Autodesk Inventor part; units mm, degrees
ref_plane "YZ Plane" through (0, 0, 0) normal (1, 0, 0) x (0, 1, 0)
ref_plane "XZ Plane" through (0, 0, 0) normal (0, 1, 0) x (-1, 0, 0)
ref_plane "XY Plane" through (0, 0, 0) normal (0, 0, 1) x (1, 0, 0)
sketch "Эскиз1" plane through (0, 0, 0) normal (0, 0, 1) x (1, 0, 0)
  line L0 (-5, -1.0438) -> (49.0851, -1.0438)
  circle A0 centre (141.53, 31.3) radius 1.6
  circle A1 centre (141.53, 31.3) radius 12.8551
  line L1 (141.53, 31.3) -> (144.3584, 34.1284)
  line L2 (144.3584, 34.1284) -> (153.4483, 25.0385)
  line L3 (144.3584, 34.1284) -> (135.2685, 43.2183)
  line L4 (135.2685, 43.2183) -> (132.4401, 40.3899)
  line L5 (133.8543, 41.8041) -> (152.0341, 23.6243)
  line L6 (152.0341, 23.6243) -> (153.4483, 25.0385)
  circle A2 centre (141.53, 31.3) radius 3.5
  line L7 (133.8543, 41.8041) -> (138.2527, 30.0714)
  line L8 (141.53, 31.3) -> (150.6199, 22.2101)
  line L9 (150.6199, 22.2101) -> (153.4483, 19.3817)
  circle A3 centre (153.4483, 19.3817) radius 1.6
  circle A4 centre (153.4483, 19.3817) radius 3.5
  line L10 (139.0551, 28.8251) -> (150.9734, 16.9068)
  line L11 (153.4483, 25.0385) -> (156.198, 21.5472)
  ellipse E0 centre (50.75, 20.1064) end of major axis (50.75, -5.3184) minor radius 3 (49.0851, -1.0438) -> (50.4608, -5.2) ccw
  line L12 (-5, -9.3562) -> (-5, -1.0438)
  line L13 (49.0851, -9.3562) -> (-5, -9.3562)
  ellipse E1 centre (50.75, -30.5064) end of major axis (50.75, -5.0816) minor radius 3 (50.4608, -5.2) -> (49.0851, -9.3562) ccw
  line L14 (135.2688, -53.6185) -> (153.4482, -35.4383)
  line L15 (153.4482, -35.4383) -> (156.1979, -31.9467)
  arc A5 (156.1979, -31.9467) -> (150.9733, -27.3065) centre (153.4482, -29.7813) ccw
  line L16 (150.9733, -27.3065) -> (139.0551, -39.2252)
  arc A6 (139.0551, -39.2252) -> (138.2526, -40.4715) centre (141.5299, -41.7001) ccw
  line L17 (138.2526, -40.4715) -> (133.8546, -52.2043)
  line L18 (133.8546, -52.2043) -> (135.2688, -53.6185)
  circle A7 centre (153.4482, -29.7813) radius 1.6
  circle A8 centre (141.5299, -41.7001) radius 1.6
  arc A9 (133.5218, -22.9864) -> (138.03, -21.6481) centre (141.53, -41.7) ccw
  arc A10 (138.03, -25.2121) -> (137.4201, -25.3535) centre (141.5299, -41.7001) ccw
  line L19 (137.4201, -25.3535) -> (133.5218, -22.9864)
  line L20 (138.03, -21.6481) -> (138.03, -25.2121)
  point P0 (0, 0)
  point P1 (139.0604, -39.2199)
  point P2 (144.9752, 30.6832)
  point P3 (140.9132, 34.7452)
  point P4 (133.9107, 41.6537)
  point P5 (135.7198, 42.7671)
  dimension "d0" = 3.2
  dimension "d1" = 4
  dimension "d2" = 7
  dimension "d3" = 4
  dimension "d4" = 3.2
  dimension "d5" = 7
extrude "Выдавливание1" add sketch "Эскиз1" against normal blind 12 contours A0 L1 L5 A2 L8 | A0 L8 A2 L5 L1 | L5 A2 L1 | L1 A2 L5 | L8 A1 L10 A2 | A2 L5 A1 L8 | A2 L5 A1 L3 L1 | L1 L2 A1 L5 A2 | A2 L7 A1 L5 | L9 A4 L10 A1 | A1 L5 L6 L11 A4 L9 | L5 L4 L3 A1 | A1 L7 L5 | A1 L2 L6 L5 | A4
chamfer "Фаска1" distance 1 angle 45 2 edges at (151.8483, 19.3817, -12) (139.93, 31.3, -12)
sketch "Эскиз2" plane through (153.4483, 25.0385, 0) normal (0.7071068, 0.7071068, 0) x (0, 0, -1)
  line L0 (0, 25.7101) -> (12, 25.7101)
  line L1 (6, 25.7101) -> (6, 21.4051)
  line L2 (6, 21.4051) -> (6, -7.5)
  line L3 (0, -7.5) -> (12, -7.5)
  line L4 (6, 21.4051) -> (6, 1.9051)
  circle A0 centre (6, 21.4051) radius 1.6
  circle A1 centre (6, 1.9051) radius 1.6
  point P0 (0, 90.7994)
  dimension "d11" = 4.305
  dimension "d12" = 19.5
  dimension "d13" = 3.2
  dimension "d14" = 3.2
extrude "Выдавливание2" [suppressed]
chamfer "Фаска2" [suppressed]
sketch "Эскиз3" plane through (139.0551, 28.8251, -12) normal (-0.7071068, -0.7071068, 0) x (0, 0, 1)
  circle A0 centre (6, -10.9499) radius 1.6
  line L0 (6, -10.9499) -> (8.7, -10.9499)
  line L1 (8.7, -12.5088) -> (6, -14.0676)
  line L2 (6, -14.0676) -> (3.3, -12.5088)
  line L3 (3.3, -12.5088) -> (3.3, -9.3911)
  line L4 (3.3, -9.3911) -> (6, -7.8323)
  line L5 (6, -7.8323) -> (8.7, -9.3911)
  line L6 (8.7, -9.3911) -> (8.7, -12.5088)
  point P0 (12, 77.9444)
  dimension "d20" = 2.7
extrude "Выдавливание3" cut sketch "Эскиз3" against normal blind 1.5
sketch "Эскиз4" plane through (139.0551, 28.8251, -12) normal (-0.7071068, -0.7071068, 0) x (0, 0, 1)
  circle A0 centre (6, 8.5501) radius 1.6
  line L0 (6, 8.5501) -> (8.7, 8.5501)
  line L1 (12, -12.8551) -> (12, 12.2169)
  line L2 (8.7, 6.9912) -> (6, 5.4324)
  line L3 (6, 5.4324) -> (3.3, 6.9912)
  line L4 (3.3, 6.9912) -> (3.3, 10.1089)
  line L5 (3.3, 10.1089) -> (6, 11.6677)
  line L6 (6, 11.6677) -> (8.7, 10.1089)
  line L7 (8.7, 10.1089) -> (8.7, 6.9912)
  point P0 (12, 77.9444)
  point P1 (12, 12.8551)
  point P2 (6, 8.5501)
  dimension "d23" = 2.7
extrude "Выдавливание4" cut sketch "Эскиз4" against normal blind 5
properties part number "laser_krepl_right"
Check sheet for the modelled part. Datum: model origin and axes. Units: mm. A direction names the side the tool comes from. Give positions to 0.01 mm unless a question says otherwise; leave off trailing zeros. Order: outer loops, then holes, each group sorted by start corner. A loop starts at its lowest first (then second) coordinate and runs counter-clockwise, first axis right, second up. Notation, with made-up numbers: M 82,-36.75 L 140,-36.75 A12 cw 140,-28.75 Z; hole C -17,13 d8. An arc over 180 degrees is marked long. Answer in a Markdown table with one row per item. Add a question column.
Q1. Sectioned sample at B-B, the plane z = -1. Record the boundary of the cut face in (x, y).
Q2. Sectioned sample at C-C, the plane y = 31.3. Record the boundary of the cut face in (x, z).
Q3. Thickness scan on L1, parallel to Z at x = 136.5, y = 38.25; L2, parallel to X at y = 31.3, z = -8.5; L3, parallel to Y at x = 147, z = -4.75. Record the ranges inside material, lowest first.
Q4. Release check for a two-part mould opening along Z. For faces 3 (the flat face through (144.231, 34.256, -5.916)), 4 (the flat face through (144, 29, 0)), 5 (the flat face through (134.81, 39.72, -7.67)) record: released by +Z, released by -Z, zero draft, split by the parting line, or undercut.
Q5. Sectioned sample at A-A, the plane x = 141.53. Record the boundary of the cut face in (y, z), and give its area (3 significant figures).
Q6. Access from +Z, -Z, +X, -X, +Y, -Y to the whole of each face (thin tool, end or side, straight path). Record for faces 1 (the flat face through (147, 22, -3.3)), 2 (the flat face through (135.506, 37.399, -5.978)).
Q7. Gauge pin test, flat ends, axial feed: pin 1 Ø1 at (x, z) = (142, -8.5) entering from -Y; pin 2 Ø2 at (y, z) = (36, -6) entering from +X; pin 3 Ø3 at (x, z) = (144, -5) entering from -Y. Record the tip position at first contact, or that the pin passes through.
Q8. Sectioned sample at D-D, the plane y = 28. Record the boundary of the cut face in (x, z).
Verdict:
| question | item | result |
|---|---|---|
| 1 | outline | M 133.85,41.8 L 138.25,30.07 A3.5 ccw 139.06,28.83 L 150.97,16.91 A3.5 ccw 156.2,21.55 L 153.45,25.04 L 135.27,43.22 Z; hole C 141.53,31.3 d3.2; hole C 153.45,19.38 d3.2 |
| 2 | outline | M 137.79,-12 L 138.93,-12 L 139.93,-11 L 139.93,0 L 137.79,0 Z; M 143.13,-11 L 144.13,-12 L 147.19,-12 L 147.19,0 L 143.13,0 Z |
| 3 | L1 | -12 to -8.7, -7.6 to -4.4, -3.3 to 0 |
| 3 | L2 | 137.79 to 139.93, 143.13 to 147.19 |
| 3 | L3 | 20.88 to 22.7, 23 to 31.49 |
| 4 | face 3 | zero draft |
| 4 | face 4 | released by +Z |
| 4 | face 5 | undercut |
| 5 | outline | M 26.35,-12 L 28.7,-12 L 29.7,-11 L 29.7,0 L 26.35,0 Z; M 32.9,-11 L 33.9,-12 L 36.96,-12 L 36.96,0 L 32.9,0 Z |
| 5 | area | 87.9 mm² |
| 6 | face 1 | none |
| 6 | face 2 | +Z, -Z, -X, -Y |
| 7 | pin 1 | y = 25.38 |
| 7 | pin 2 | x = 143.49 |
| 7 | pin 3 | y = 22.58 |
| 8 | outline | M 139.88,-12 L 150.49,-12 L 150.49,0 L 139.88,0 Z |
